from build123d import *

# Parameters (mm, degrees)
F0_W     = 26.75
F0_H     = 26.75
F1_DEPTH = 2500
F2_W     = 26.75
F2_H     = 50
F2_H_2   = 40
F3_DEPTH = 2.5


with BuildPart() as f1:
    # F0 (on Top) → F1 (new body)
    with BuildSketch(Plane.XY):
        with BuildLine():
            ThreePointArc((15.875, 13.375), (15.142766953, 15.142766953), (13.375, 15.875))
            Line((13.375, 15.875), (-13.375, 15.875))
            ThreePointArc((-13.375, 15.875), (-15.142766953, 15.142766953), (-15.875, 13.375))
            Line((-15.875, 13.375), (-15.875, -13.375))
            ThreePointArc((-15.875, -13.375), (-15.142766953, -15.142766953), (-13.375, -15.875))
            Line((-13.375, -15.875), (13.375, -15.875))
            ThreePointArc((13.375, -15.875), (15.142766953, -15.142766953), (15.875, -13.375))
            Line((15.875, -13.375), (15.875, 13.375))
        make_face()
        Rectangle(F0_W, F0_H, mode=Mode.SUBTRACT)
    extrude(amount=F1_DEPTH)

    # F2 (on face) → F3 (join)
    with BuildSketch(Plane.XZ.offset(15.875)):
        with Locations((0, 2515)):
            Rectangle(F2_W, F2_H)
        with Locations((0, -10)):
            Rectangle(F2_W, F2_H_2)
    extrude(amount=F3_DEPTH)

    # F4: F1 across plane


with BuildPart() as f1_1:
    add(f1.part)
    add(f1.part.mirror(Plane.XZ))


solid = f1_1.part
Verification items for the finished model (mm, model axes). Coordinates: 2 decimals unless noted, no trailing zeros. Loops run counter-clockwise (first coordinate to the right, second up) from the corner with the lowest first, then second, coordinate; pieces in that order, holes last. Notation, with made-up numbers: (-3.5, 58.5) -> (34.5, 58.5) arc R30 ccw to (34.5, 81.5) -> close; hole circle Ø7 at (80.5, -12). An arc over 180 degrees is marked (long way). Write each question's results on one line, items separated by ' | '.
Item 1: Section check C-C, the plane z = 1736. Enter the section's corners in (x, y) (3 decimals).
Found:
outline: (-15.875, -13.375) arc R2.5 ccw to (-13.375, -15.875) -> (13.375, -15.875) arc R2.5 ccw to (15.875, -13.375) -> (15.875, 13.375) arc R2.5 ccw to (13.375, 15.875) -> (-13.375, 15.875) arc R2.5 ccw to (-15.875, 13.375) -> close; hole (-13.375, -13.375) -> (13.375, -13.375) -> (13.375, 13.375) -> (-13.375, 13.375) -> close
Item 2: Section check A-A, the plane y = 4. Enter the section's corners in (x, z) (3 decimals).
Found:
outline: (-15.875, 0) -> (-13.375, 0) -> (-13.375, 2500) -> (-15.875, 2500) -> close; (13.375, 0) -> (15.875, 0) -> (15.875, 2500) -> (13.375, 2500) -> close
Item 3: Gauge pin test, flat ends, axial feed: pin 1 (3 mm diameter, centred on y = -17, z = 2517.5, fed in from +X) (3 decimals); pin 2 (1 mm diameter, centred on x = -2.5, y = 12, fed in from +Z); pin 3 (3 mm diameter, centred on y = -17.5, z = -6, fed in from -X) (3 decimals); pin 4 (8 mm diameter, centred on x = 11.5, z = 864, fed in from -Y) (3 decimals). Record the tip position at first contact, or that the pin passes through.
Found:
pin 1: stops at x = 13.375 | pin 2: passes through | pin 3: stops at x = -13.375 | pin 4: stops at y = -15.875
Item 4: Section check B-B, the plane x = 6.5. Enter the section's corners in (y, z) (3 decimals).
Found:
outline: (-18.375, -30) -> (-15.875, -30) -> (-15.875, 0) -> (-13.375, 0) -> (-13.375, 2500) -> (-15.875, 2500) -> (-15.875, 2540) -> (-18.375, 2540) -> (-18.375, 2490) -> (-15.875, 2490) -> (-15.875, 10) -> (-18.375, 10) -> close; (13.375, 0) -> (15.875, 0) -> (15.875, -30) -> (18.375, -30) -> (18.375, 10) -> (15.875, 10) -> (15.875, 2490) -> (18.375, 2490) -> (18.375, 2540) -> (15.875, 2540) -> (15.875, 2500) -> (13.375, 2500) -> close
Item 5: Material ranges on L1, parallel to Y at x = 7, z = 1293 (3 decimals); L2, parallel to X at y = 13.5, z = 1399, recorded low to high.
Found:
L1: y = -15.875 to -13.375, 13.375 to 15.875 | L2: x = -15.87 to 15.87
